Design review of the part shown in the three views and the two pictorial views. Dimensions are in mm from the part's minimum x, y and z. A direction names the side the tool comes from. Coordinates: 2 decimals unless noted, no trailing zeros. Loops run counter-clockwise (first coordinate to the right, second up) from the corner with the lowest first, then second, coordinate; pieces in that order, holes last. Notation, with made-up numbers: (13.25, -13) -> (24.25, -13) arc R16 ccw to (24.25, 9) -> close; hole circle Ø2 at (-15.75, 28.5). An arc over 180 degrees is marked (long way). Use a Markdown table: item, result. Add a question column.
Q1. Take a section at A-A on y = 34.5. Write out the cut boundary in (x, z), plus the area to 3 significant figures.
Q2. Take a section at D-D on x = 11.5. Write out the cut boundary in (y, z), plus the area to 3 significant figures.
Q3. Clearance check with flat-ended pins moving along their axes: pin 1 Ø5 at (x, z) = (37, 9) entering from +Y; pin 2 Ø8 at (x, z) = (36.5, 15) entering from +Y; pin 3 Ø15 at (x, y) = (22.5, 10) entering from +Z; pin 4 Ø4 at (x, y) = (36, 36.5) entering from -Z. State where each tip first meets the part, or that it passes through.
Q4. For the marked faces 1, 2, 3, 4 and 5, list the 3-axis set-ups (+Z, -Z, +X, -X, +Y, -Y) from which the entire face can be reached by the end or side of a thin tool; tool diameter is ignored.
Q5. Take a section at C-C on y = 7. Write out the cut boundary in (x, z), plus the area to 3 significant figures.
Q6. Take a section at B-B on z = 9. Write out the cut boundary in (x, y).
Q7. For probe 1 along X at (y, z) = (35.5, 6); probe 2 along Z at (x, y) = (31, 29.5); probe 3 along Z at (x, y) = (5, 12.5), list the stretches that pass through material, from the lowest coordinate up.
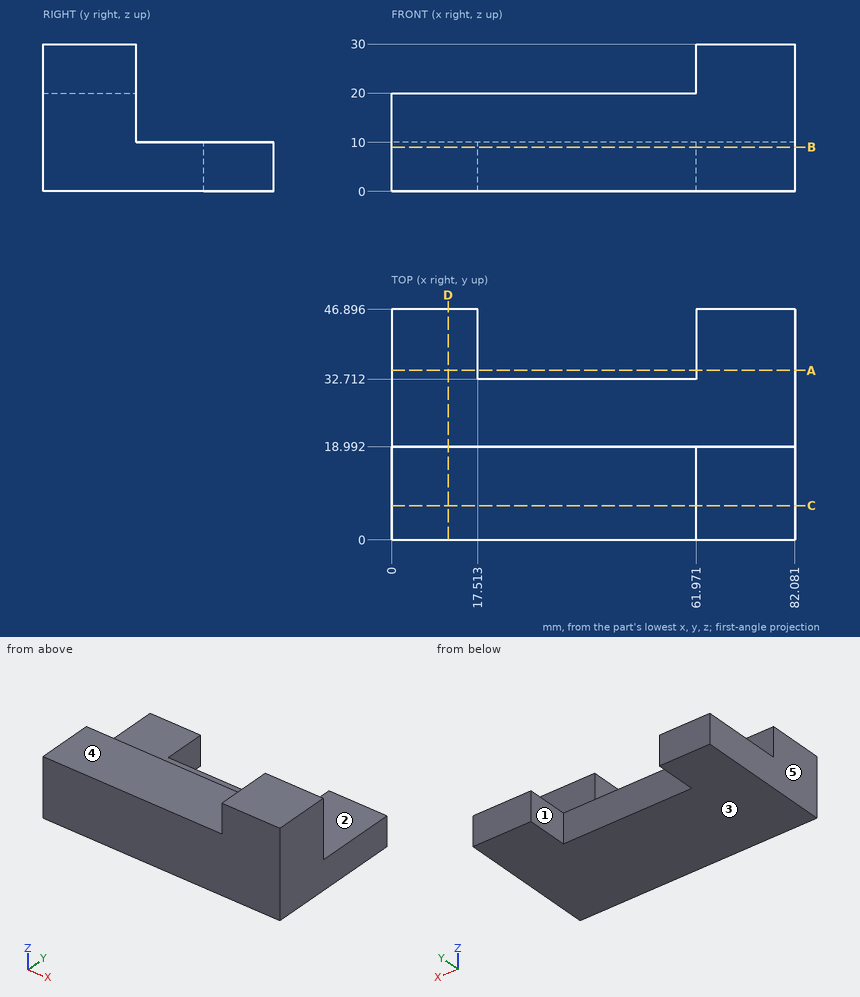
Answer list:
| question | item | result |
|---|---|---|
| 1 | outline | (0, 0) -> (17.51, 0) -> (17.51, 10) -> (0, 10) -> close; (61.97, 0) -> (82.08, 0) -> (82.08, 10) -> (61.97, 10) -> close |
| 1 | area | 376 mm² |
| 2 | outline | (0, 0) -> (46.9, 0) -> (46.9, 10) -> (18.99, 10) -> (18.99, 20) -> (0, 20) -> close |
| 2 | area | 659 mm² |
| 3 | pin 1 | y = 32.71 |
| 3 | pin 2 | y = 18.99 |
| 3 | pin 3 | z = 20 |
| 3 | pin 4 | through |
| 4 | face 1 | +Z, -Z, +Y |
| 4 | face 2 | +Z, +X, -X, +Y |
| 4 | face 3 | -Z, +X, -X, +Y, -Y |
| 4 | face 4 | +Z, -X, +Y, -Y |
| 4 | face 5 | +Z, -Z, -X, +Y, -Y |
| 5 | outline | (0, 0) -> (82.08, 0) -> (82.08, 30) -> (61.97, 30) -> (61.97, 20) -> (0, 20) -> close |
| 5 | area | 1,840 mm² |
| 6 | outline | (0, 0) -> (82.08, 0) -> (82.08, 46.9) -> (61.97, 46.9) -> (61.97, 32.71) -> (17.51, 32.71) -> (17.51, 46.9) -> (0, 46.9) -> close |
| 7 | probe 1 | 0 to 17.51, 61.97 to 82.08 |
| 7 | probe 2 | 0 to 10 |
| 7 | probe 3 | 0 to 20 |
